Verification items for the finished model (mm, model axes). Face numbers are marked on the shaded views. A direction names the side the tool comes from. Give positions to 0.01 mm unless a question says otherwise; leave off trailing zeros. Order: outer loops, then holes, each group sorted by start corner. A loop starts at its lowest first (then second) coordinate and runs counter-clockwise, first axis right, second up. Notation, with made-up numbers: (17.5, -15) -> (33.5, -15) arc R14 cw to (33.5, 9) -> close; hole circle Ø6 at (31.25, 61.5). An arc over 180 degrees is marked (long way). Write each question's results on one line, items separated by ' | '. Start each with the question number.
1. Cross-section at A-A, the plane x = -5. Enter the section's corners in (y, z), then the cut area to 3 significant figures.
2. Cross-section at C-C, the plane y = -6.5. Enter the section's corners in (x, z).
3. Set-up check for the marked faces 4 and 5: record each of +Z, -Z, +X, -X, +Y, -Y from which the full face is reachable in a straight line by a thin tool's end or side.
4. Depth check by flat-ended pin: pin 1 Ø2 at (x, y) = (-2, 8.5) entering from -Z. Enter the tip coordinate at first touch or a pass-through.
5. Mould release check, pull along Y, two halves, no side actions. Record for the marked faces 1, 2 and 3: +Y half, -Y half, draft (parallel to the pull), parting line (faces both ways), or undercut.
6. Cross-section at B-B, the plane z = 5.25. Enter the section's corners in (x, y), then the cut area to 3 significant figures.
7. Material ranges on L1, parallel to Y at x = -4.5, z = 2.5; L2, parallel to Z at x = 0, y = -15.3; L3, parallel to X at y = -15.25, z = 3.25, recorded low to high. Write a range as from..to.
from build123d import *

# Parameters (mm, degrees)
SKETCH2_W                 = 29.487
SKETCH2_H                 = 26
BOSS_EXTRUDE1_DEPTH       = 6.5
CUT_EXTRUDE1_DEPTH        = 23.623473849
M2X0_4_TAPPED_HOLE1_D     = 1.6
M2X0_4_TAPPED_HOLE1_DEPTH = 5.2
M2X0_4_TAPPED_HOLE1_TIP   = 0.480688495


with BuildPart() as part:
    # Sketch2 → Boss-Extrude1 (new body)
    with BuildSketch(Plane(origin=(0, 0, 0), x_dir=(0, 1, 0), z_dir=(0, 0, 1))):
        with Locations((-2.5935, 0)):
            Rectangle(SKETCH2_W, SKETCH2_H)
    extrude(amount=BOSS_EXTRUDE1_DEPTH)

    # Sketch1 → Cut-Extrude1 (cut, through all)
    with BuildSketch(Plane(origin=(0, 0, 0), x_dir=(0, 1, 0), z_dir=(0, 0, 1))):
        with BuildLine():
            Line((-9.15, 7.917543811), (-9.15, -7.917543811))
            ThreePointArc((-9.15, -7.917543811), (0, -12.1), (9.15, -7.917543811))
            Line((9.15, -7.917543811), (9.15, 7.917543811))
            ThreePointArc((9.15, 7.917543811), (0, 12.1), (-9.15, 7.917543811))
        make_face()
    extrude(amount=CUT_EXTRUDE1_DEPTH, mode=Mode.SUBTRACT)

    # M2x0.4 Tapped Hole1
    with Locations(Plane.XZ.offset(17.337)):
        with Locations((0, 3.25)):
            Hole(M2X0_4_TAPPED_HOLE1_D / 2, depth=M2X0_4_TAPPED_HOLE1_DEPTH)
            with Locations((0, 0, -(M2X0_4_TAPPED_HOLE1_DEPTH + M2X0_4_TAPPED_HOLE1_TIP / 2))):  # 118° drill point
                Cone(0, M2X0_4_TAPPED_HOLE1_D / 2, M2X0_4_TAPPED_HOLE1_TIP, mode=Mode.SUBTRACT)


solid = part.part
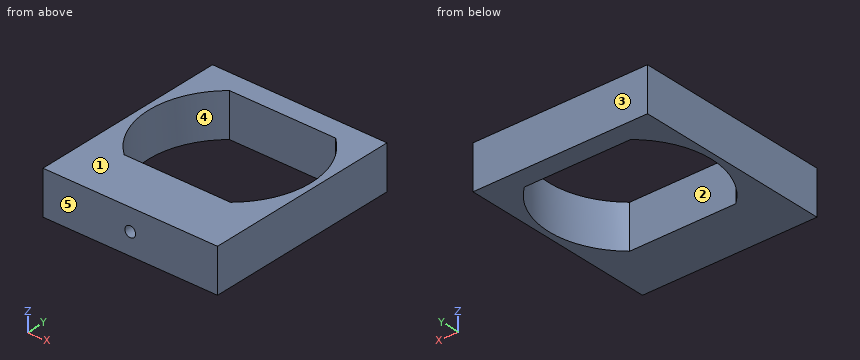
Results below:
1) outline: (-17.34, 0) -> (-9.15, 0) -> (-9.15, 6.5) -> (-17.34, 6.5) -> close; (9.15, 0) -> (12.15, 0) -> (12.15, 6.5) -> (9.15, 6.5) -> close | area: 72.7 mm²
2) outline: (-13, 0) -> (-10.21, 0) -> (-10.21, 6.5) -> (-13, 6.5) -> close; (10.21, 0) -> (13, 0) -> (13, 6.5) -> (10.21, 6.5) -> close
3) face 4: +Z, -Z | face 5: +Z, -Z, +X, -X, -Y
4) pin 1: stops at z = 0
5) face 1: draft | face 2: undercut | face 3: +Y half
6) outline: (-13, -17.34) -> (13, -17.34) -> (13, 12.15) -> (-13, 12.15) -> close; hole (-7.92, -9.15) -> (7.92, -9.15) arc R12.1 ccw to (7.92, 9.15) -> (-7.92, 9.15) arc R12.1 ccw to start | area: 371 mm²
7) L1: y = -17.34..-9.15, 9.15..12.15 | L2: z = 0..2.45, 4.05..6.5 | L3: x = -13..-0.8, 0.8..13
